Input: part model. Units: mm. Frame: model coordinates. Give positions to 0.01 mm unless a question says otherwise; leave off trailing zeros. Loops run counter-clockwise (first coordinate to the right, second up) from the corner with the lowest first, then second, coordinate; pieces in that order, holes last. Notation, with made-up numbers: (63.5, 81.5) - (97.5, 81.5) arc R18 cw to (97.5, 100.5) - close; hole circle Ø3 at (65.5, 37.25). An arc over 180 degrees is marked (long way). Answer as a JSON object with one key per item and string values. Group by question number.
(1) Material intervals for L1, parallel to X at y = -4.5, z = -4.1; L2, parallel to Z at x = 11, y = 1.75; L3, parallel to X at y = 8.5, z = -0.5, sorted ascending.
(2) Pin query (flat end, axial travel): P1, Ø0.7, axis at x = 0, z = -3, coming from the +Y side; P2, Ø8, axis at x = 4.5, y = -10, coming from the +Z side; P3, Ø1.5, axis at y = 9.5, z = -4, coming from the +X side; P4, Ø1.5, axis at x = 0.5, z = -1, coming from the -Y side. Return the tip coordinate at first contact, or that it passes through.
(3) Section query A-A (z = -4.1). Return loops of the section in (x, y), plus the area to 3 significant figures.
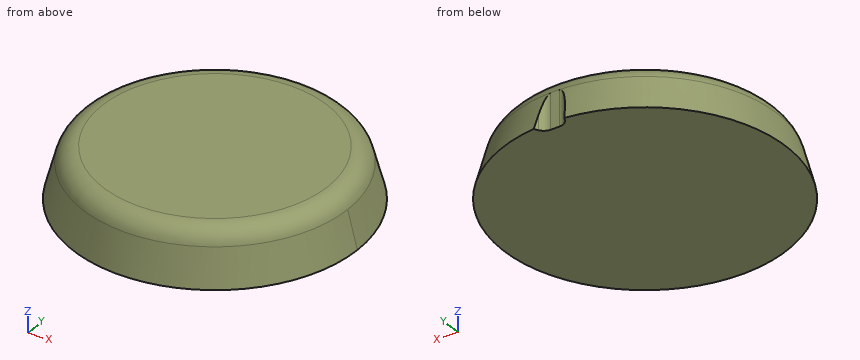
```python
from build123d import *
from build123d import SkipClean  # not in build123d's __all__

# Parameters (mm, degrees)
F0_R     = 12.5
F1_DEPTH = 5
F1_TAPER = -15
F2_R     = 2
F4_DEPTH = 25
F5_R     = 1


with BuildPart() as f1:
    # F0 (on Top) → F1 (new body)
    with BuildSketch(Plane.XY):
        Circle(F0_R)
    extrude(amount=-F1_DEPTH, taper=F1_TAPER)

    # F2
    f2_edges = [f1.edges().sort_by_distance(p)[0] for p in [
        (-12.5, 0, 0),
    ]]
    fillet(f2_edges, radius=F2_R)

    # F3 (on Top) → F4 (cut)
    with BuildSketch(Plane.XY):
        with BuildLine():
            ThreePointArc((1.5, 13.7582182094), (0, 13.8397459622), (-1.5, 13.7582182094))
            Line((-1.5, 13.7582182094), (-1, 12.8971976766))
            Line((-1, 12.8971976766), (1, 12.8971976766))
            Line((1, 12.8971976766), (1.5, 13.7582182094))
        make_face()
    with SkipClean():  # cleaning this boolean's faces spoils the solid; the shape is the same uncleaned
        extrude(amount=-F4_DEPTH, mode=Mode.SUBTRACT)

    # F5
    f5_edges = [f1.edges().sort_by_distance(p)[0] for p in [
        (-1, 12.897198, -3.313415),
        (1, 12.897198, -3.313415),
    ]]
    fillet(f5_edges, radius=F5_R)


solid = f1.part
```
Recorded:
{
 "1": {"L1": "x = -12.83 to 12.83", "L2": "z = -5 to -0.01", "L3": "x = -8.87 to 8.87"},
 "2": {"P1": "stops at y = 12.9", "P2": "stops at z = 0", "P3": "stops at x = 10.43", "P4": "stops at y = -12.96"},
 "3": {"outline": "(-1.37, 13.53) arc R13.6 ccw (long way) to (1.37, 13.53) - (1.29, 13.4) arc R1 cw to (0.42, 12.9) - (-0.42, 12.9) arc R1 cw to (-1.29, 13.4) - close", "area": "579 mm^2"}
}
